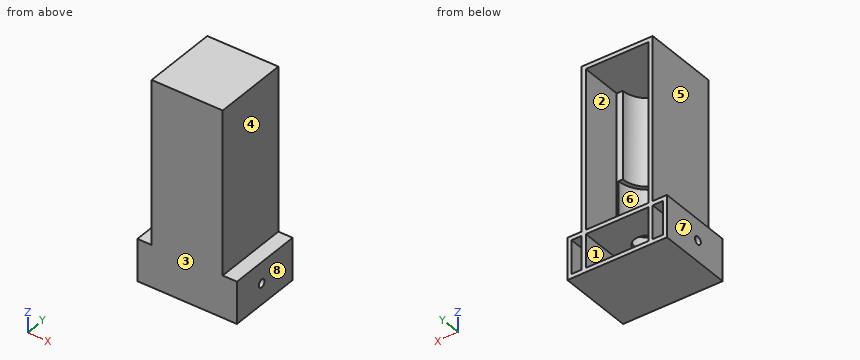
```python
from build123d import *

# Parameters (mm, degrees)
BOSS_EXTRUDE1_DEPTH      = 12.7
SKETCH2_W                = 53.879496
SKETCH2_H                = 57.15
BOSS_EXTRUDE2_DEPTH      = 3.175
CUT_EXTRUDE2_DEPTH       = 66.145131417
CUT_EXTRUDE2_DEPTH_BACK  = 66.145131417
SKETCH3_R                = 3
SKETCH5_W                = 53.879496
SKETCH5_H                = 25.4
SKETCH5_R                = 3.4925
BOSS_EXTRUDE3_DEPTH      = 6.35
SKETCH7_W                = 7.62
SKETCH7_H                = 15.609396712
BOSS_EXTRUDE7_DEPTH      = 1.5875
SKETCH8_W                = 53.879496
SKETCH8_H                = 57.15
BOSS_EXTRUDE8_DEPTH      = 127
CUT_EXTRUDE7_DEPTH       = 154.323065852
CUT_EXTRUDE7_DEPTH_BACK  = 154.323065852
SKETCH13_W               = 0.002356984
SKETCH13_H               = 124.229061331
CUT_EXTRUDE8_START       = -31.75
SKETCH14_W               = 47.527139016
SKETCH14_H               = 120.65
CUT_EXTRUDE8_DEPTH       = 31.75
CUT_EXTRUDE9_DEPTH       = 4.229066359
SKETCH16_W               = 53.879496
SKETCH16_H               = 25.4
CUT_EXTRUDE10_DEPTH      = 152.071109158
SKETCH18_W               = 13.97
SKETCH18_H               = 31.75
SKETCH18_W_2             = 7.62
SKETCH18_H_2             = 25.4
BOSS_EXTRUDE10_DEPTH     = 57.15
BOSS_EXTRUDE11_START     = -34.559748
BOSS_EXTRUDE11_DEPTH     = 7.62
BOSS_EXTRUDE12_START     = 26.939748
BOSS_EXTRUDE12_DEPTH     = 7.62
CUT_EXTRUDE11_DEPTH      = 163.985890519
CUT_EXTRUDE11_DEPTH_BACK = 163.985890519
SKETCH20_R               = 3


with BuildPart() as part:
    # Sketch1 → Boss-Extrude1 (new, symmetric)
    with BuildSketch(Plane.XY):
        Polygon((-26.939748, 0), (26.939748, 0), (26.939748, 6.35), (26.939748, 57.15), (23.764748, 57.15), (23.764748, 6.35), (-23.764748, 6.35), (-23.764748, 57.15), (-26.939748, 57.15), (-26.939748, 6.35), align=None)
    extrude(amount=BOSS_EXTRUDE1_DEPTH, both=True)

    # Sketch2 → Boss-Extrude2 (add)
    with BuildSketch(Plane(origin=(0, 0, -12.7), x_dir=(-1, 0, 0), z_dir=(0, 0, -1))):
        with Locations((0, 28.575)):
            Rectangle(SKETCH2_W, SKETCH2_H)
    extrude(amount=BOSS_EXTRUDE2_DEPTH)

    # Sketch6 → Revolve2 (revolve)
    with BuildSketch(Plane.XY, mode=Mode.PRIVATE) as revolve2_sk:
        Polygon((-23.764748, 25.4), (-16.144748, 25.4), (-16.144748, 30.48), (-21.224748, 30.48), (-23.764748, 33.02), align=None)
        Polygon((23.764748, 33.02), (23.764748, 25.4), (16.144748, 25.4), (16.144748, 30.48), (21.224748, 30.48), align=None)
    revolve(revolve2_sk.sketch.rotate(Axis((-23.764748, 25.4, 0), (1, 0, 0)), 90), axis=Axis((-23.764748, 25.4, 0), (1, 0, 0)))

    # Sketch3 → Cut-Extrude2 (cut, two sides: drawn at the far end of the back side and taken through both)
    with BuildSketch(Plane(origin=(0, 0, 0), x_dir=(0, 0, -1), z_dir=(1, 0, 0)).offset(-CUT_EXTRUDE2_DEPTH_BACK)):
        with Locations((0, 25.4)):
            Circle(SKETCH3_R)
    extrude(amount=CUT_EXTRUDE2_DEPTH + CUT_EXTRUDE2_DEPTH_BACK, mode=Mode.SUBTRACT)

    # Sketch5 → Boss-Extrude3 (add)
    with BuildSketch(Plane.XZ):
        with Locations((0, -28.575)):
            Rectangle(SKETCH5_W, SKETCH5_H)
        with Locations(Location((7.889748, -28.575, 0), (0, 0, 270))):
            Circle(SKETCH5_R, mode=Mode.SUBTRACT)
        with Locations(Location((-17.510252, -28.575, 0), (0, 0, 270))):
            Circle(SKETCH5_R, mode=Mode.SUBTRACT)
    extrude(amount=-BOSS_EXTRUDE3_DEPTH)

    # Sketch7 → Boss-Extrude7 (add, symmetric)
    with BuildSketch(Plane.XY):
        with Locations((-19.954748, 14.154698356)):
            Rectangle(SKETCH7_W, SKETCH7_H)
        with Locations((19.954748, 14.154698356)):
            Rectangle(SKETCH7_W, SKETCH7_H)
    extrude(amount=BOSS_EXTRUDE7_DEPTH, both=True)

    # Sketch8 → Boss-Extrude8 (add)
    with BuildSketch(Plane.XY.offset(12.7)):
        with Locations((0, 28.575)):
            Rectangle(SKETCH8_W, SKETCH8_H)
    extrude(amount=BOSS_EXTRUDE8_DEPTH)

    # Sketch9 → Cut-Revolve1 (revolve, cut)
    with BuildSketch(Plane(origin=(0, 0, 0), x_dir=(0, 0, -1), z_dir=(1, 0, 0))):
        Polygon((-70.104, 47.752), (-70.104, 44.577), (-136.525, 44.577), (-136.525, 25.4), (-70.104, 25.4), (0, 25.4), (0, 35.56), (-20.104066359, 35.56), (-20.104066359, 44.577), (-32.004, 44.577), (-32.004, 47.752), align=None)
    revolve(axis=Axis((0, 25.4, 0), (0, 0, 1)), mode=Mode.SUBTRACT)

    # Sketch13 → Cut-Extrude7 (cut, two sides: drawn at the far end of the back side and taken through both)
    with BuildSketch(Plane(origin=(0, 0, 0), x_dir=(-1, 0, 0), z_dir=(0, -1, 0)).offset(-CUT_EXTRUDE7_DEPTH_BACK)):
        with Locations((26.940926492, -77.585469335)):
            Rectangle(SKETCH13_W, SKETCH13_H)
        with Locations((-26.938569508, -77.585469335)):
            Rectangle(SKETCH13_W, SKETCH13_H)
    extrude(amount=CUT_EXTRUDE7_DEPTH + CUT_EXTRUDE7_DEPTH_BACK, mode=Mode.SUBTRACT)

    # Sketch14 → Cut-Extrude8 (cut)
    with BuildSketch(Plane(origin=(0, 57.15, 0), x_dir=(1, 0, 0), z_dir=(0, 1, 0)).offset(CUT_EXTRUDE8_START)):
        with Locations((-0.001178492, -76.2)):
            Rectangle(SKETCH14_W, SKETCH14_H)
    extrude(amount=CUT_EXTRUDE8_DEPTH, mode=Mode.SUBTRACT)

    # Sketch15 → Cut-Extrude9 (cut)
    with BuildSketch(Plane.XY.offset(20.104066359)):
        with BuildLine():
            Line((-10.16, 25.4), (-19.177, 25.4))
            ThreePointArc((-19.177, 25.4), (0, 6.223), (19.177, 25.4))
            Line((19.177, 25.4), (10.16, 25.4))
            ThreePointArc((10.16, 25.4), (0, 15.24), (-10.16, 25.4))
        make_face()
    extrude(amount=-CUT_EXTRUDE9_DEPTH, mode=Mode.SUBTRACT)

    # Sketch16 → Cut-Extrude10 (cut, through all)
    with BuildSketch(Plane(origin=(0, 6.35, 0), x_dir=(1, 0, 0), z_dir=(0, 1, 0))):
        with Locations((0, 28.575)):
            Rectangle(SKETCH16_W, SKETCH16_H)
    extrude(amount=-CUT_EXTRUDE10_DEPTH, mode=Mode.SUBTRACT)

    # Sketch18 → Boss-Extrude10 (add)
    with BuildSketch(Plane(origin=(0, 0, 0), x_dir=(1, 0, 0), z_dir=(0, 1, 0))):
        with Locations((-30.749748, 0)):
            Rectangle(SKETCH18_W, SKETCH18_H)
        with Locations((-30.749748, 0)):
            Rectangle(SKETCH18_W_2, SKETCH18_H_2, mode=Mode.SUBTRACT)
    boss_extrude10 = extrude(amount=BOSS_EXTRUDE10_DEPTH)

    # Sketch19 → Boss-Extrude11 (add)
    with BuildSketch(Plane(origin=(0, 0, 0), x_dir=(0, 0, -1), z_dir=(1, 0, 0)).offset(BOSS_EXTRUDE11_START)):
        with BuildLine():
            Line((1.5875, 22.854446278), (12.7, 29.784605952))
            Line((12.7, 29.784605952), (12.7, 0))
            Line((12.7, 0), (-12.7, 0))
            Line((-12.7, 0), (-12.7, 29.784605952))
            Line((-12.7, 29.784605952), (-1.5875, 22.854446278))
            ThreePointArc((-1.5875, 22.854446278), (0, 22.4), (1.5875, 22.854446278))
        make_face()
    extrude(amount=BOSS_EXTRUDE11_DEPTH)

    # Mirror4: Boss-Extrude10 across plane
    add(boss_extrude10.mirror(Plane(origin=(0, 0, 0), x_dir=(0, 0, 1), z_dir=(1, 0, 0))))

    # Sketch19<2> → Boss-Extrude12 (add)
    with BuildSketch(Plane(origin=(0, 0, 0), x_dir=(0, 0, -1), z_dir=(1, 0, 0)).offset(BOSS_EXTRUDE12_START)):
        with BuildLine():
            Line((1.5875, 22.854446278), (12.7, 29.784605952))
            Line((12.7, 29.784605952), (12.7, 0))
            Line((12.7, 0), (-12.7, 0))
            Line((-12.7, 0), (-12.7, 29.784605952))
            Line((-12.7, 29.784605952), (-1.5875, 22.854446278))
            ThreePointArc((-1.5875, 22.854446278), (0, 22.4), (1.5875, 22.854446278))
        make_face()
    extrude(amount=BOSS_EXTRUDE12_DEPTH)

    # Sketch20 → Cut-Extrude11 (cut, two sides: drawn at the far end of the back side and taken through both)
    with BuildSketch(Plane(origin=(-23.764748, 0, 0), x_dir=(0, 0, -1), z_dir=(1, 0, 0)).offset(-CUT_EXTRUDE11_DEPTH_BACK)):
        with Locations((0, 25.4)):
            Circle(SKETCH20_R)
    extrude(amount=CUT_EXTRUDE11_DEPTH + CUT_EXTRUDE11_DEPTH_BACK, mode=Mode.SUBTRACT)


solid = part.part
```
Source: CAD feature listing. Evaluate the final solid. Frame: model axes, mm. Face numbers are marked on the shaded views. A direction names the side the tool comes from. Give positions to 0.01 mm unless a question says otherwise; leave off trailing zeros. Write each loop counter-clockwise with the first axis right and the second up, starting at its lowest first coordinate (ties: lowest second). Pieces come first, ordered by that corner, then holes.
1. Material intervals for line 1 along X through (y, z) = (54, -6); line 2 along X through (y, z) = (16.5, 4); line 3 along X through (y, z) = (40.5, 107), sorted ascending.
2. Pull-direction query (Y, two-part tool) for the marked faces 1, 2 and 3; classes: +Y half, -Y half, draft (parallel to the pull), parting line (faces both ways), or undercut.
3. Section query C-C (y = 50). Return the cut outline in (x, z) (3 decimals).
4. First-contact query: pin 1 (3 mm diameter, centred on x = 30, y = 20.5, fed in from +Z) (3 decimals); pin 2 (12.5 mm diameter, centred on x = -2, z = 3, fed in from +Y); pin 3 (6 mm diameter, centred on y = 30, z = 96.5, fed in from -X). Flat tips, straight axial feed; report the tip coordinate or a pass-through.
5. Section query B-B (x = 0). Return the cut outline in (y, z) (3 decimals).
6. Section query D-D (z = 100.5). Return the cut outline in (x, y).
7. Section query A-A (z = 0). Count the separate pieces of the cut face and the enclosed holes in it, then the cut area to 3 significant figures.
8. Access query for the marked faces 4, 5, 6, 7 and 8. Directions: +Z, -Z, +X, -X, +Y, -Y. A direction counts if a zero-diameter tool reaches every point of the face in a straight line with its end or side. Return the directions, or none.
Output values:
1. line 1: x = -37.73 to -34.56, -26.94 to -23.76, 23.76 to 26.94, 34.56 to 37.73
1. line 2: x = -37.73 to -23.76, 23.76 to 37.73
1. line 3: x = -26.94 to -23.76, 23.76 to 26.94
2. face 1: undercut
2. face 2: draft
2. face 3: -Y half
3. outline: (-37.735, -15.875) - (37.735, -15.875) - (37.735, 15.875) - (26.937, 15.875) - (26.937, 139.7) - (-26.94, 139.7) - (-26.94, 15.875) - (-37.735, 15.875) - close; hole (-34.56, -12.7) - (-26.94, -12.7) - (-26.94, 12.7) - (-34.56, 12.7) - close; hole (-23.765, -12.7) - (23.765, -12.7) - (23.765, 12.7) - (-23.765, 12.7) - close; hole (-23.765, 15.875) - (23.762, 15.875) - (23.762, 136.525) - (-23.765, 136.525) - close; hole (26.94, -12.7) - (34.56, -12.7) - (34.56, 12.7) - (26.94, 12.7) - close
4. pin 1: stops at z = 15.875
4. pin 2: stops at y = 6.35
4. pin 3: stops at x = -26.94
5. outline: (0, -15.875) - (57.15, -15.875) - (57.15, -12.7) - (6.35, -12.7) - (6.35, 12.7) - (15.24, 12.7) - (15.24, 15.875) - (6.223, 15.875) - (6.223, 32.004) - (3.048, 32.004) - (3.048, 70.104) - (6.223, 70.104) - (6.223, 136.525) - (57.15, 136.525) - (57.15, 139.7) - (0, 139.7) - close; (35.56, 12.7) - (57.15, 12.7) - (57.15, 15.875) - (35.56, 15.875) - close
6. outline: (-26.94, 0) - (26.94, 0) - (26.94, 57.15) - (23.76, 57.15) - (23.76, 25.4) - (19.18, 25.4) arc R19.18 cw to (-19.18, 25.4) - (-23.76, 25.4) - (-23.76, 57.15) - (-26.94, 57.15) - close
7. separate pieces: 5
7. enclosed holes: 0
7. area: 1,580 mm2
8. face 4: +Z, +X, +Y, -Y
8. face 5: +Z, -X, +Y, -Y
8. face 6: +Y
8. face 7: +Z, -Z, -X, +Y, -Y
8. face 8: +Z, -Z, +X, +Y, -Y
